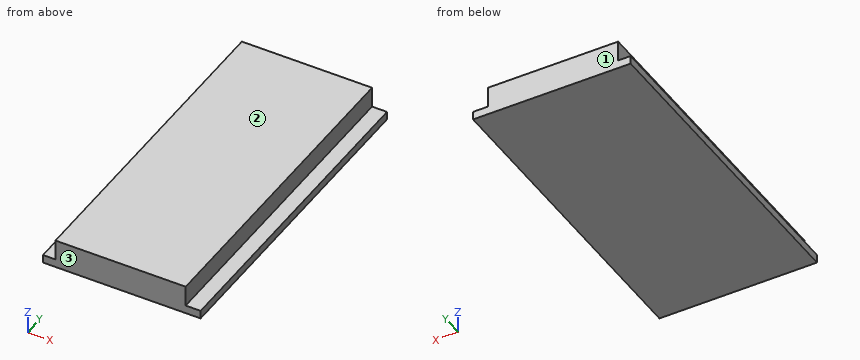
from build123d import *

# Parameters (mm, degrees)
BOX004_W     = 15.7
BOX004_H     = 39
BOX004_DEPTH = 3.5
BOX003_W     = 19
BOX003_H     = 39
BOX003_DEPTH = 1


with BuildPart() as cubo004:
    # Box004 → Box004 (new body)
    with BuildSketch(Plane(origin=(1.5, -14, 0), x_dir=(1, 0, 0), z_dir=(0, 0, 1))):
        with Locations((7.85, 19.5)):
            Rectangle(BOX004_W, BOX004_H)
    extrude(amount=BOX004_DEPTH)


with BuildPart() as fusion001:
    # Box003 → Box003 (new body)
    with BuildSketch(Plane(origin=(0, -14, 0), x_dir=(1, 0, 0), z_dir=(0, 0, 1))):
        with Locations((9.5, 19.5)):
            Rectangle(BOX003_W, BOX003_H)
    extrude(amount=BOX003_DEPTH)

    # Fusion001: union Cubo004
    add(cubo004.part)


solid = fusion001.part
Verification items for the finished model (mm, model axes). Face numbers are marked on the shaded views. Give positions to 0.01 mm unless a question says otherwise; leave off trailing zeros. Order: outer loops, then holes, each group sorted by start corner. A loop starts at its lowest first (then second) coordinate and runs counter-clockwise, first axis right, second up. Notation, with made-up numbers: M 41.5,87.5 L 61.5,87.5 A23 cw 61.5,116.5 Z; hole C 86,34 d5. An arc over 180 degrees is marked long. Use one line per item in the form item = value. Start each with the question number.
Q1. Scan line: line 1 along X through (y, z) = (15, 2.15). Record every from-to range of solid material in increasing order. Write a range as [from, to].
Q2. Mould release check, pull along Y, two halves, no side actions. Record for the marked faces 1, 2 and 3: +Y half, -Y half, draft (parallel to the pull), parting line (faces both ways), or undercut.
Q3. Section check A-A (y = 11). Enter the section's corners in (x, z).
Q4. Go/stop test with flat-tipped pins: pin 1 Ø2 at (y, z) = (14, 2.5) entering from -X; pin 2 Ø1.2 at (x, y) = (0.5, 2) entering from +Z; pin 3 Ø1.2 at (y, z) = (1.5, 2.5) entering from +X. Record where each tip stops, or that it passes through.
Q5. Section check B-B (z = 2.7). Enter the section's corners in (x, y).
Evaluation:
q1.line_1 = [1.5, 17.2]
q2.face_1 = +Y half
q2.face_2 = draft
q2.face_3 = -Y half
q3.outline = M 0,0 L 19,0 L 19,1 L 17.2,1 L 17.2,3.5 L 1.5,3.5 L 1.5,1 L 0,1 Z
q4.pin_1 = 1.5
q4.pin_2 = 1
q4.pin_3 = 17.2
q5.outline = M 1.5,-14 L 17.2,-14 L 17.2,25 L 1.5,25 Z
